Source: CAD feature listing. Evaluate the final solid. Frame: model axes, mm. A direction names the side the tool comes from. Give positions to 0.01 mm unless a question says otherwise; leave off trailing zeros. Loops run counter-clockwise (first coordinate to the right, second up) from the corner with the lowest first, then second, coordinate; pieces in that order, holes last. Notation, with made-up numbers: M 17,23.25 L 25,23.25 A15 cw 25,45.25 Z; hole C -1,61 d3. An arc over 180 degrees is marked long. Put each result on its own line as item: value.
from build123d import *

# Parameters (mm, degrees)
SKETCH_2_R                   = 183
EXTRUDE_1_DEPTH              = 7.75
HOLE_WIZARD_M5_1_D           = 5.5
HOLE_WIZARD_M5_1_CBORE_D     = 9
HOLE_WIZARD_M5_1_CBORE_DEPTH = 6
SKETCH_6_W                   = 499.91157149
SKETCH_6_H                   = 215.35218654
CUT_EXTRUDE_1_DEPTH          = 267.151754372
EXTRUDE_2_DEPTH              = 427
SKETCH_8_W                   = 538.874028387
SKETCH_8_H                   = 388.77669628
CUT_EXTRUDE_2_DEPTH          = 467.660847956
HOLE_WIZARD_1_D              = 5.5
HOLE_WIZARD_1_CBORE_D        = 10
HOLE_WIZARD_1_CBORE_DEPTH    = 5.7


with BuildPart() as part:
    # 草图1 → 旋转1 (revolve)
    with BuildSketch(Plane.XY, mode=Mode.PRIVATE) as revolve_1_sk:
        with BuildLine():
            Line((185.156666985, 2.25), (0, 2.25))
            Line((0, 2.25), (0, -2.25))
            Line((0, -2.25), (185.156666985, -2.25))
            Line((185.156666985, -2.25), (187.78506482, -0.409576022))
            add(Edge.make_bspline(
                [(187.78506482, 0.409576022), (187.830906121, 0.377477598), (187.871837762, 0.337021948), (187.904470176, 0.291559224), (187.937102589, 0.246096499), (187.962335818, 0.194372782), (187.978080287, 0.140671335), (187.993824756, 0.086969887), (188.000514717, 0.029809558), (187.997596172, -0.026076181), (187.994677627, -0.08196192), (187.982070079, -0.138114466), (187.960817564, -0.189883804), (187.939565048, -0.241653142), (187.909081396, -0.290467133), (187.87189097, -0.332283469), (187.846140091, -0.361237358), (187.816805619, -0.387350876), (187.78506482, -0.409576022)],
                knots=[0, 0, 0, 0, 0.000167886, 0.000167886, 0.000167886, 0.000335771, 0.000335771, 0.000335771, 0.000503657, 0.000503657, 0.000503657, 0.000671543, 0.000671543, 0.000671543, 0.000839428, 0.000839428, 0.000839428, 0.000954806, 0.000954806, 0.000954806, 0.000954806], degree=3))
            Line((187.78506482, 0.409576022), (185.156666985, 2.25))
        make_face()
    revolve(revolve_1_sk.sketch.rotate(Axis((0, 2.25, 0), (0, -1, 0)), 270), axis=Axis((0, 2.25, 0), (0, -1, 0)))

    # 草图2 → 凸台-拉伸1 (add)
    with BuildSketch(Plane.XZ.offset(2.25)):
        with Locations(Location((0, 0, 0), (0, 0, 270))):
            Circle(SKETCH_2_R)
    extrude(amount=EXTRUDE_1_DEPTH)

    # 草图3 → 切除-旋转1 (revolve, cut)
    with BuildSketch(Plane.XY, mode=Mode.PRIVATE) as cut_revolve_1_sk:
        with BuildLine():
            Line((165.843333015, 2.25), (0, 2.25))
            Line((0, 2.25), (0, -10))
            Line((0, -10), (168, -10))
            Line((168, -10), (168, -2.25))
            Line((168, -2.25), (165.843333015, -2.25))
            Line((165.843333015, -2.25), (163.21493518, -0.409576022))
            ThreePointArc((163.21493518, -0.409576022), (163.001723398, 0), (163.21493518, 0.409576022))
            Line((163.21493518, 0.409576022), (165.843333015, 2.25))
        make_face()
    revolve(cut_revolve_1_sk.sketch.rotate(Axis((0, 2.25, 0), (0, -1, 0)), 270), axis=Axis((0, 2.25, 0), (0, -1, 0)), mode=Mode.SUBTRACT)

    # M5 六角头螺栓的柱形沉头孔1 (through all)
    with Locations(Plane(origin=(0, 2.25, 0), x_dir=(1, 0, 0), z_dir=(0, 1, 0))):
        with Locations((-45.422742415, -169.519982514), (-124.097240098, -124.097240098), (-169.519982514, -45.422742415), (45.422742415, -169.519982514), (124.097240098, -124.097240098), (169.519982514, -45.422742415), (-45.422742415, 169.519982514), (-124.097240098, 124.097240098), (-169.519982514, 45.422742415), (45.422742415, 169.519982514), (124.097240098, 124.097240098), (169.519982514, 45.422742415)):
            CounterBoreHole(HOLE_WIZARD_M5_1_D / 2, HOLE_WIZARD_M5_1_CBORE_D / 2, HOLE_WIZARD_M5_1_CBORE_DEPTH)

    # 草图6 → 切除-拉伸1 (cut, through all)
    with BuildSketch(Plane(origin=(0, 2.25, 0), x_dir=(1, 0, 0), z_dir=(0, 1, 0))):
        with Locations((-5.153727541, -107.67609327)):
            Rectangle(SKETCH_6_W, SKETCH_6_H)
    extrude(amount=-CUT_EXTRUDE_1_DEPTH, mode=Mode.SUBTRACT)

    # 草图7 → 凸台-拉伸2 (add)
    with BuildSketch(Plane.XY):
        with BuildLine():
            Line((-185.156666985, 2.25), (-187.78506482, 0.409576022))
            add(Edge.make_bspline(
                [(-187.78506482, 0.409576022), (-187.830906121, 0.377477598), (-187.871837762, 0.337021948), (-187.904470176, 0.291559224), (-187.937102589, 0.246096499), (-187.962335818, 0.194372782), (-187.978080287, 0.140671335), (-187.993824756, 0.086969887), (-188.000514717, 0.029809558), (-187.997596172, -0.026076181), (-187.994677627, -0.08196192), (-187.982070079, -0.138114466), (-187.960817564, -0.189883804), (-187.939565048, -0.241653142), (-187.909081396, -0.290467133), (-187.87189097, -0.332283469), (-187.846140091, -0.361237358), (-187.816805619, -0.387350876), (-187.78506482, -0.409576022)],
                knots=[0, 0, 0, 0, 0.000167886, 0.000167886, 0.000167886, 0.000335771, 0.000335771, 0.000335771, 0.000503657, 0.000503657, 0.000503657, 0.000671543, 0.000671543, 0.000671543, 0.000839428, 0.000839428, 0.000839428, 0.000954806, 0.000954806, 0.000954806, 0.000954806], degree=3))
            Line((-187.78506482, -0.409576022), (-185.156666985, -2.25))
            Line((-185.156666985, -2.25), (-183, -2.25))
            Line((-183, -2.25), (-183, -10))
            Line((-183, -10), (-168, -10))
            Line((-168, -10), (-168, -2.25))
            Line((-168, -2.25), (-165.843333015, -2.25))
            Line((-165.843333015, -2.25), (-163.21493518, -0.409576022))
            ThreePointArc((-163.21493518, -0.409576022), (-163.001723398, 0), (-163.21493518, 0.409576022))
            Line((-163.21493518, 0.409576022), (-165.843333015, 2.25))
            Line((-165.843333015, 2.25), (-185.156666985, 2.25))
        make_face()
    extrude(amount=EXTRUDE_2_DEPTH)

    # 草图8 → 切除-拉伸2 (cut, through all)
    with BuildSketch(Plane.XY):
        with Locations((39.369792029, -22.329590013)):
            Rectangle(SKETCH_8_W, SKETCH_8_H)
    extrude(amount=-CUT_EXTRUDE_2_DEPTH, mode=Mode.SUBTRACT)

    # 打孔尺寸(%根据)内六角圆柱头螺钉的类型1 (through all)
    with Locations(Plane(origin=(0, 2.25, 0), x_dir=(1, 0, 0), z_dir=(0, 1, 0))):
        with Locations((-175.5, -50), (-175.5, -450), (-175.5, -150), (-175.5, -350), (-175.5, -250)):
            CounterBoreHole(HOLE_WIZARD_1_D / 2, HOLE_WIZARD_1_CBORE_D / 2, HOLE_WIZARD_1_CBORE_DEPTH)


solid = part.part
1. Material intervals for line 1 (Z direction, x = -175.5, y = 0.25); line 2 (Z direction, x = -175.5, y = -6); line 3 (X direction, y = -6.25, z = 250), sorted ascending. Write a range as from..to.
Found:
line 1: 0..45, 55..145, 155..245, 255..345, 355..427
line 2: 0..47.25, 52.75..147.25, 152.75..247.25, 252.75..347.25, 352.75..427
line 3: -183..-178.25, -172.75..-168
2. Access query for faces 1 (the flat face through (-176, -2, 427)), 2 (the cylindrical face through (-179.185, -0.56, 46.621)). Directions: +Z, -Z, +X, -X, +Y, -Y. A direction counts if a zero-diameter tool reaches every point of the face in a straight line with its end or side. Return the directions, or none.
Found:
face 1: +Z, +X, -X, +Y, -Y
face 2: +Y
3. Draft query along X for faces 3 (the cylindrical face through (-179.5, -0.6, 153)), 4 (the flat face through (-175, 2.25, 211)), 5 (the flat face through (-183, -6, 211)), 6 (the flat face through (-168, -6, 211)). Return one class per face: pulls with the +X half, pulls with the -X half, needs draft (parallel to the pull), parting line crosses it, or undercut.
Found:
face 3: undercut
face 4: needs draft
face 5: pulls with the -X half
face 6: pulls with the +X half
4. Contact query for flat-ended pins moving along their axis: P1, Ø1, axis at x = -167, z = 304.5, coming from the -Y side; P2, Ø9, axis at x = -175.5, z = 250, coming from the +Y side; P3, Ø6, axis at y = -4.5, z = 307, coming from the +X side. Output: stop coordinate, or through.
Found:
P1: y = -2.25
P2: y = -3.45
P3: x = -164.77
5. Section query A-A (y = -6.75). Output: boundary loops of the cut face in (x, z), plus the area to 3 significant figures.
Found:
outline: M -183,0 L -168,0 L -168,427 L -183,427 Z; hole C -175.5,50 d5.5; hole C -175.5,150 d5.5; hole C -175.5,250 d5.5; hole C -175.5,350 d5.5
area: 6,310 mm^2
